For this review, use the dimensioned drawing (mm, ordinates from the lowest corner) and the shaded views. A direction names the side the tool comes from. Round coordinates to 2 decimals unless told otherwise and drop trailing zeros. Order: outer loops, then holes, each group sorted by start corner. A loop starts at its lowest first (then second) coordinate and runs counter-clockwise, first axis right, second up. Notation, with made-up numbers: (-33.75, -9) -> (4.25, -9) arc R30 cw to (4.25, 21) -> close; hole circle Ø8 at (-12, 34.25). An arc over 180 degrees is marked (long way). Answer in a Markdown table with one row per item.
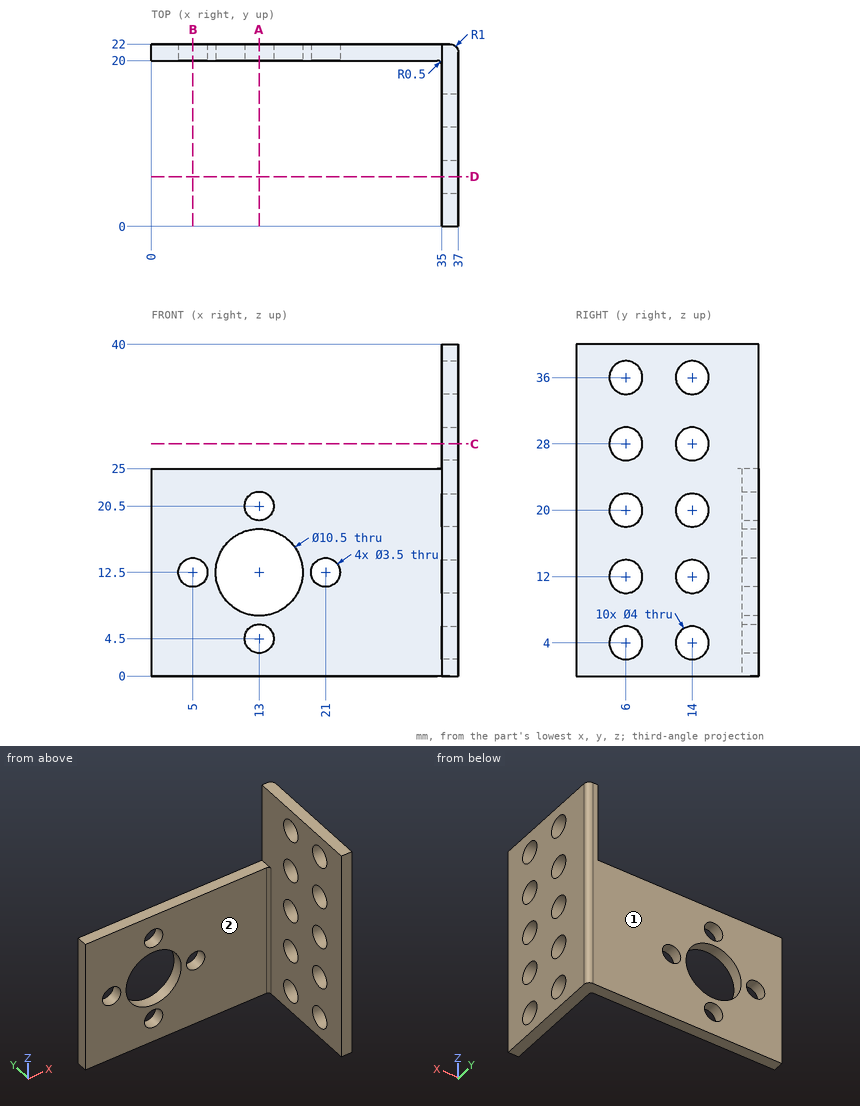
Q1. Tool access review of the marked faces 1 and 2: name each direction out of +Z, -Z, +X, -X, +Y, -Y from which nothing blocks a thin tool from reaching the whole face with its end or side.
Answer key:
| item | result |
|---|---|
| face 1 | +Z, -Z, +X, -X, +Y |
| face 2 | +Z, -Z, -X, -Y |
Q2. Take a section at B-B, the plane x = 5. Write out the cut boundary in (y, z).
Answer key:
| item | result |
|---|---|
| outline | (20, 0) -> (22, 0) -> (22, 10.75) -> (20, 10.75) -> close; (20, 14.25) -> (22, 14.25) -> (22, 25) -> (20, 25) -> close |
Q3. Clearance check with flat-ended pins moving along their axes: pin 1 Ø6.5 at (y, z) = (6, 20) entering from +X; pin 2 Ø1.2 at (x, y) = (16.5, 20) entering from +Z; pin 3 Ø20 at (x, z) = (9.5, 7.5) entering from -Y; pin 4 Ø2 at (y, z) = (16, 21) entering from -X. State where each tip first meets the part, or that it passes through.
Answer key:
| item | result |
|---|---|
| pin 1 | stops at x = 37 |
| pin 2 | stops at z = 25 |
| pin 3 | stops at y = 20 |
| pin 4 | stops at x = 35 |
Q4. Take a section at A-A, the plane x = 13. Write out the cut boundary in (y, z), then the cut area to 3 significant figures.
Answer key:
| item | result |
|---|---|
| outline | (20, 0) -> (22, 0) -> (22, 2.75) -> (20, 2.75) -> close; (20, 6.25) -> (22, 6.25) -> (22, 7.25) -> (20, 7.25) -> close; (20, 17.75) -> (22, 17.75) -> (22, 18.75) -> (20, 18.75) -> close; (20, 22.25) -> (22, 22.25) -> (22, 25) -> (20, 25) -> close |
| area | 15.0 mm^2 |
Q5. Take a section at C-C, the plane z = 28. Write out the cut boundary in (x, y), then the cut area to 3 significant figures.
Answer key:
| item | result |
|---|---|
| outline | (35, 0) -> (37, 0) -> (37, 4) -> (35, 4) -> close; (35, 8) -> (37, 8) -> (37, 12) -> (35, 12) -> close; (35, 16) -> (37, 16) -> (37, 21) arc R1 ccw to (36, 22) -> (35, 22) -> close |
| area | 27.8 mm^2 |
Q6. To check wall thickness, follow probe 1 along Y at (x, z) = (36.1, 20); probe 2 along X at (y, z) = (20.8, 20.5); probe 3 along X at (y, z) = (5.75, 22.5). State the ranges of each line that lie inside material, in increasing order.
Answer key:
| item | result |
|---|---|
| probe 1 | y = 0 to 4, 8 to 12, 16 to 21.99 |
| probe 2 | x = 0 to 11.25, 14.75 to 37 |
| probe 3 | x = 35 to 37 |
Q7. Take a section at D-D, the plane y = 6. Write out the cut boundary in (x, z), then the cut area to 3 significant figures.
Answer key:
| item | result |
|---|---|
| outline | (35, 0) -> (37, 0) -> (37, 2) -> (35, 2) -> close; (35, 6) -> (37, 6) -> (37, 10) -> (35, 10) -> close; (35, 14) -> (37, 14) -> (37, 18) -> (35, 18) -> close; (35, 22) -> (37, 22) -> (37, 26) -> (35, 26) -> close; (35, 30) -> (37, 30) -> (37, 34) -> (35, 34) -> close; (35, 38) -> (37, 38) -> (37, 40) -> (35, 40) -> close |
| area | 40.0 mm^2 |
